Geometry check sheet. Reference: the model listing, model coordinates, mm. A direction names the side the tool comes from. Give positions to 0.01 mm unless a question says otherwise; leave off trailing zeros. Loops run counter-clockwise (first coordinate to the right, second up) from the corner with the lowest first, then second, coordinate; pieces in that order, holes last.
```python
from build123d import *

# Parameters (mm, degrees)
BASEHEAD_DEPTH = 4.7752


with BuildPart() as part:
    # Sketch1 → BaseHead (new body)
    with BuildSketch(Plane(origin=(0, 0, 0), x_dir=(0, 0, -1), z_dir=(1, 0, 0))):
        Polygon((5.5626, 3.211568607), (5.5626, -3.211568607), (0, -6.423137215), (-5.5626, -3.211568607), (-5.5626, 3.211568607), (0, 6.423137215), align=None)
    extrude(amount=BASEHEAD_DEPTH)

    # BodySke → BaseBody (revolve)
    with BuildSketch(Plane.XY):
        Polygon((0, 0), (68.2752, 0), (68.2752, 2.41935), (67.51955, 3.175), (0, 3.175), align=None)
    revolve(axis=Axis((0, 0, 0), (1, 0, 0)))

    # Sketch3 → HeadChamfer (revolve, cut)
    with BuildSketch(Plane.XY):
        Polygon((0, 5.5626), (4.163005602, 12.773137215), (4.163005602, 19.123137215), (-12.7, 19.123137215), (-12.7, 5.5626), align=None)
    revolve(axis=Axis((0, 0, 0), (1, 0, 0)), mode=Mode.SUBTRACT)


solid = part.part
```
1) Depth check by flat-ended pin: P1, Ø6, axis at x = 8, y = 1.5, coming from the -Z side (3 decimals); P2, Ø5, axis at x = 18.5, y = -4, coming from the -Z side; P3, Ø4, axis at x = 56.5, z = -3, coming from the +Y side. Enter the tip coordinate at first touch or a pass-through.
2) Tool access check on faces 1 (the flat face through (2, 0, -5.563)), 2 (the cylindrical face through (35.71, -0.69, -3.1)). Record the directions out of +Z, -Z, +X, -X, +Y, -Y that give a thin tool (end or side, any length) a straight path to the whole face; none if there is none.
3) Scan lines: line 1 along X through (y, z) = (-0.25, -4.75); line 2 along Z through (x, y) = (55.5, 0.5); line 3 along Y through (x, z) = (8, 1.25). Record each from-to range of solid material in increasing order.
4) Sectioned sample at A-A on x = 25.5. Enter the section's corners in (y, z) (3 decimals), plus the area to 3 significant figures.
Determined:
1. P1: stops at z = -3.175
1. P2: stops at z = -2.8
1. P3: stops at y = 3.01
2. face 1: -Z, +X, -X, +Y, -Y
2. face 2: +X
3. line 1: x = 0 to 4.78
3. line 2: z = -3.14 to 3.14
3. line 3: y = -2.92 to 2.92
4. outline: circle Ø6.35 at (0, 0)
4. area: 31.7 mm2
